from build123d import *

# Parameters (mm, degrees)
SKETCH1_R           = 22.86
BOSS_EXTRUDE1_DEPTH = 44.45
SKETCH2_R           = 3.175
BOSS_EXTRUDE2_DEPTH = 25.4
CUT_EXTRUDE1_DEPTH  = 7.62
FILLET1_R           = 2.286
SKETCH4_R           = 2.54
BOSS_EXTRUDE3_DEPTH = 6.35


with BuildPart() as part:
    # Sketch1 → Boss-Extrude1 (new body)
    with BuildSketch(Plane.XY):
        Circle(SKETCH1_R)
    extrude(amount=BOSS_EXTRUDE1_DEPTH)

    # Sketch2 → Boss-Extrude2 (add)
    with BuildSketch(Plane.XY.offset(44.45)):
        Circle(SKETCH2_R)
    extrude(amount=BOSS_EXTRUDE2_DEPTH)

    # Sketch3 → Cut-Extrude1 (cut)
    with BuildSketch(Plane.XY.offset(44.45)):
        with BuildLine():
            Line((13.413435382, 0), (15.953435382, 0))
            ThreePointArc((15.953435382, 0), (13.816080318, 7.976717691), (7.976717691, 13.816080318))
            Line((7.976717691, 13.816080318), (6.706717691, 11.616375793))
            ThreePointArc((6.706717691, 11.616375793), (11.616375793, 6.706717691), (13.413435382, 0))
        make_face()
        with BuildLine():
            Line((9.246717691, 16.015784844), (10.516717691, 18.215489369))
            ThreePointArc((10.516717691, 18.215489369), (18.215489369, 10.516717691), (21.033435382, 0))
            Line((21.033435382, 0), (18.493435382, 0))
            ThreePointArc((18.493435382, 0), (16.015784844, 9.246717691), (9.246717691, 16.015784844))
        make_face()
        with BuildLine():
            Line((11.616375793, -6.706717691), (13.816080318, -7.976717691))
            ThreePointArc((13.816080318, -7.976717691), (7.976717691, -13.816080318), (0, -15.953435382))
            Line((0, -15.953435382), (0, -13.413435382))
            ThreePointArc((0, -13.413435382), (6.706717691, -11.616375793), (11.616375793, -6.706717691))
        make_face()
        with BuildLine():
            Line((16.015784844, -9.246717691), (18.215489369, -10.516717691))
            ThreePointArc((18.215489369, -10.516717691), (10.516717691, -18.215489369), (0, -21.033435382))
            Line((0, -21.033435382), (0, -18.493435382))
            ThreePointArc((0, -18.493435382), (9.246717691, -16.015784844), (16.015784844, -9.246717691))
        make_face()
        with BuildLine():
            Line((-6.706717691, -11.616375793), (-7.976717691, -13.816080318))
            ThreePointArc((-7.976717691, -13.816080318), (-13.816080318, -7.976717691), (-15.953435382, 0))
            Line((-15.953435382, 0), (-13.413435382, 0))
            ThreePointArc((-13.413435382, 0), (-11.616375793, -6.706717691), (-6.706717691, -11.616375793))
        make_face()
        with BuildLine():
            Line((-9.246717691, -16.015784844), (-10.516717691, -18.215489369))
            ThreePointArc((-10.516717691, -18.215489369), (-18.215489369, -10.516717691), (-21.033435382, 0))
            Line((-21.033435382, 0), (-18.493435382, 0))
            ThreePointArc((-18.493435382, 0), (-16.015784844, -9.246717691), (-9.246717691, -16.015784844))
        make_face()
        with BuildLine():
            Line((-11.616375793, 6.706717691), (-13.816080318, 7.976717691))
            ThreePointArc((-13.816080318, 7.976717691), (-7.976717691, 13.816080318), (0, 15.953435382))
            Line((0, 15.953435382), (0, 13.413435382))
            ThreePointArc((0, 13.413435382), (-6.706717691, 11.616375793), (-11.616375793, 6.706717691))
        make_face()
        with BuildLine():
            Line((-16.015784844, 9.246717691), (-18.215489369, 10.516717691))
            ThreePointArc((-18.215489369, 10.516717691), (-10.516717691, 18.215489369), (0, 21.033435382))
            Line((0, 21.033435382), (0, 18.493435382))
            ThreePointArc((0, 18.493435382), (-9.246717691, 16.015784844), (-16.015784844, 9.246717691))
        make_face()
    extrude(amount=-CUT_EXTRUDE1_DEPTH, mode=Mode.SUBTRACT)

    # Fillet1
    # the kernel refuses this fillet: 2.286 mm, written as the material it takes off along each edge
    with BuildSketch(Plane(origin=(0, 0, 44.45), x_dir=(1, 0, 0), z_dir=(0, -1, 0))) as fillet1_piece_1:
        with BuildLine():
            CenterArc((22.86 - FILLET1_R, -FILLET1_R), FILLET1_R, 0, 90)
            Line((22.86 - FILLET1_R, 0), (22.86, 0))
            Line((22.86, 0), (22.86, -FILLET1_R))
        make_face()
    revolve(axis=Axis((0, 0, 44.45), (0, 0, 1)), mode=Mode.SUBTRACT)

    # Sketch4 → Boss-Extrude3 (add)
    with BuildSketch(Plane(origin=(0, 0, 0), x_dir=(-1, 0, 0), z_dir=(0, 0, -1))):
        with Locations(Location((0, 0, 0), (0, 0, 180))):
            Circle(SKETCH4_R)
    extrude(amount=BOSS_EXTRUDE3_DEPTH)


solid = part.part
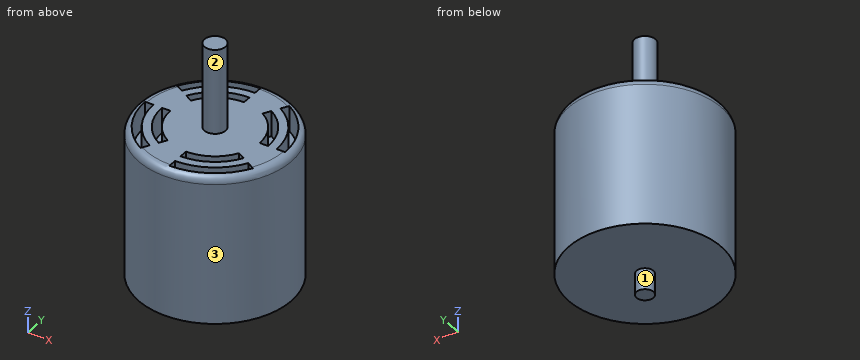
Build history of the part. All positions in model axes, mm. Face numbers are marked on the shaded views. A direction names the side the tool comes from. Coordinates: 2 decimals unless noted, no trailing zeros. Write each loop counter-clockwise with the first axis right and the second up, starting at its lowest first coordinate (ties: lowest second). Pieces come first, ordered by that corner, then holes.
(1) Cut at B-B on z = 46. List the corners of the cut face in (x, y) (3 decimals), and give its area (3 significant figures).
(2) Drill centre lines: line 1 (X direction, y = 5.5, z = 38); line 2 (Z direction, x = 8, y = -7); line 3 (Z direction, x = 13.5, y = -16). Where is each one in solid material? Low to high.
(3) 3-axis set-ups, long thin cutter, end or side, ignore diameter. For the marked faces 1, 2 and 3: which of +Z, -Z, +X, -X, +Y, -Y reach the whole face in a straight line?
(4) Pin check, flat tips, straight feed: pin 1 Ø4 at (x, y) = (14, 15.5) entering from -Z; pin 2 Ø0.8 at (x, z) = (20, 42) entering from +Y; pin 3 Ø12 at (x, z) = (11.5, 10) entering from -Y. Stop position of each tip, or through.
(5) Cut at A-A on z = 19.5. List the corners of the cut face in (x, y).
Working result:
1. outline: circle Ø6.35 at (0, 0)
1. area: 31.7 mm2
2. line 1: x = -22.19 to 12.23, 14.98 to 17.66, 20.3 to 22.19
2. line 2: z = 0 to 44.45
2. line 3: z = 0 to 36.83
3. face 1: -Z
3. face 2: +Z
3. face 3: +Z, -Z
4. pin 1: stops at z = 0
4. pin 2: stops at y = 11.77
4. pin 3: stops at y = -22.19
5. outline: circle Ø45.72 at (0, 0)
